Read the model definition and answer for the solid it produces. Units are mm, in the model's axes. Face numbers are marked on the shaded views. A direction names the side the tool comes from. Coordinates: 2 decimals unless noted, no trailing zeros. Loops run counter-clockwise (first coordinate to the right, second up) from the corner with the lowest first, then second, coordinate; pieces in that order, holes last. Notation, with made-up numbers: (52.5, 23.25) - (105.5, 23.25) arc R22 ccw to (105.5, 29.25) - close; hole circle Ø5 at (78, 70.5). An arc over 180 degrees is marked (long way). Use CSV: the item, a comma, the result in double quotes.
```python
from build123d import *

# Parameters (mm, degrees)
SKETCH2_R           = 5
SKETCH1_R           = 10
SKETCH3_W           = 28.361759846
SKETCH3_H           = 6.844946114
BOSS_EXTRUDE1_DEPTH = 10


with BuildPart() as part:
    # Sketch2 → Loft1 section 0
    with BuildSketch(Plane(origin=(0, 20, 0), x_dir=(1, 0, 0), z_dir=(0, 1, 0))):
        Circle(SKETCH2_R)
    # Sketch1 → Loft1 section 1
    with BuildSketch(Plane(origin=(0, 0, 0), x_dir=(1, 0, 0), z_dir=(0, 1, 0))):
        Circle(SKETCH1_R)
    loft()

    # Sketch3 → Boss-Extrude1 (add)
    with BuildSketch(Plane.XZ):
        Rectangle(SKETCH3_W, SKETCH3_H)
    extrude(amount=BOSS_EXTRUDE1_DEPTH)


solid = part.part
```
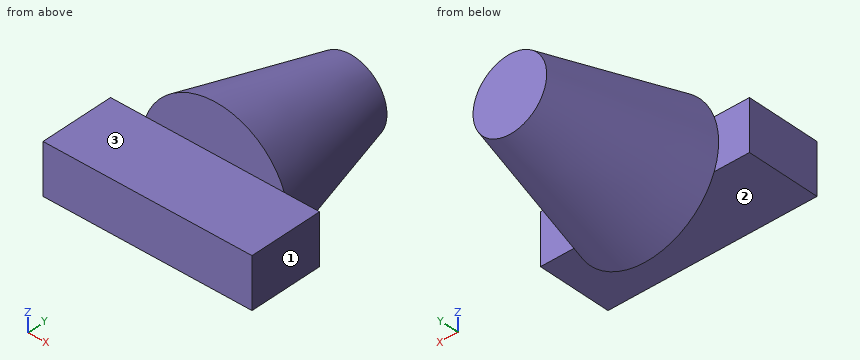
Q1. The part is cut by section C-C on x = -12.25. Determine the outline of the cut face in (y, z), and give its area (3 significant figures).
Reported:
outline,"(-10, -3.42) - (0, -3.42) - (0, 3.42) - (-10, 3.42) - close"
area,"68.4 mm²"
Q2. The part is cut by section D-D on y = 12. Determine the outline of the cut face in (x, z), and give its area (3 significant figures).
Reported:
outline,"circle Ø14 at (0, 0)"
area,"154 mm²"
Q3. A tool of negligible diameter and unlimited length cuts with its end or side. For the marked faces 1, 2 and 3, from which of +Z, -Z, +X, -X, +Y, -Y can it reach the whole face along a straight path? Write none if from no direction.
Reported:
face 1,"+Z, -Z, +X, +Y, -Y"
face 2,"-Z, +X, -X, -Y"
face 3,"+Z, +X, -X, -Y"
Q4. Given P1, Ø5.5, axis at x = -13, z = 0, coming from the +Y side; P2, Ø6, axis at y = 6.5, z = -1.5, coming from the +X side; P3, Ø3, axis at x = 1, y = -6.5, coming from the -Z side, each flat-ended and moving along its own axis, determine where each tip first touches the part or whether it passes through.
Reported:
P1,"stops at y = 0"
P2,"stops at x = 9.07"
P3,"stops at z = -3.42"
Q5. The part is cut by section B-B on y = -6. Determine the outline of the cut face in (x, z), and give its area (3 significant figures).
Reported:
outline,"(-14.18, -3.42) - (14.18, -3.42) - (14.18, 3.42) - (-14.18, 3.42) - close"
area,"194 mm²"
Q6. Find the intervals of material crossed by probe 1 along Y at (x, z) = (-2.25, -3.5); probe 2 along Y at (x, z) = (-12.5, -1); probe 3 along Z at (x, y) = (-4.5, -8), in increasing order. Write a range as [from, to].
Reported:
probe 1,"y = [0, 20]"
probe 2,"y = [-10, 0]"
probe 3,"z = [-3.42, 3.42]"
Q7. The part is cut by section A-A on x = 0. Determine the outline of the cut face in (y, z).
Reported:
outline,"(-10, -3.42) - (0, -3.42) - (0, -10) - (20, -5) - (20, 5) - (0, 10) - (0, 3.42) - (-10, 3.42) - close"
